Input: part model. Units: mm. Frame: model coordinates. Give positions to 0.01 mm unless a question says otherwise; leave off trailing zeros. Loops run counter-clockwise (first coordinate to the right, second up) from the corner with the lowest first, then second, coordinate; pieces in that order, holes last. Notation, with made-up numbers: (55, -5) - (77, -5) arc R31 cw to (77, 33) - close; hole circle Ø11 at (-38.5, 64). An arc over 180 degrees is marked (long way). One line per item, written item: value.
Autodesk Inventor part; units mm, degrees
ref_plane "YZ Plane" through (0, 0, 0) normal (1, 0, 0) x (0, 1, 0)
ref_plane "XZ Plane" through (0, 0, 0) normal (0, 1, 0) x (-1, 0, 0)
ref_plane "XY Plane" through (0, 0, 0) normal (0, 0, 1) x (1, 0, 0)
sketch "スケッチ2" plane through (0, 0, 0) normal (0, 0, 1) x (1, 0, 0)
  line L0 (-31.5, 10) -> (31.5, 10)
  line L1 (31.5, 10) -> (31.5, -10)
  line L2 (31.5, -10) -> (-31.5, -10)
  line L3 (-31.5, -10) -> (-31.5, 10)
  line L4 (0, 14) -> (0, -14) construction
  line L5 (-44.1, 0) -> (44.1, 0) construction
  point P0 (0, 0)
  dimension "d1" = 63
  dimension "d2" = 20
  dimension "d3" = 10
  dimension "d4" = 31.5
extrude "押し出し1" add sketch "スケッチ2" along normal blind 3
sketch "スケッチ3" plane through (0, 0, 3) normal (0, 0, 1) x (1, 0, 0)
  line L0 (-31.5, -10) -> (31.5, -10) construction
  line L1 (31.5, -10) -> (31.5, 10) construction
  line L2 (31.5, 10) -> (-31.5, 10) construction
  line L3 (-31.5, 10) -> (-31.5, -10) construction
  line L4 (-44.1, 0) -> (44.1, 0) construction
  point P0 (0, 0)
  point P1 (-21.5, 0)
  point P2 (1.5, 0)
  point P3 (21.5, 0)
  dimension "d7" = 10
  dimension "d8" = 10
  dimension "d9" = 20
hole "穴1" at (-21.5, 0, 3) at (1.5, 0, 3) at (21.5, 0, 3) direction (0, 0, -1) diameter 4.5 end through all
fillet "フィレット1" radius 2 4 edges at (-31.5, 10, 1.5) (31.5, 10, 1.5) (31.5, -10, 1.5) (-31.5, -10, 1.5)
equation "\"d3\" = 0.5 * d2"
equation "\"d4\" = 0.5 * d1"
properties part number "rocker_bogie_mount"
Item 1: Section B-B, the plane x = -21.5. Output: boundary loops of the cut face in (y, z), and give its area (3 significant figures).
Verdict:
outline: (-10, 0) - (-2.25, 0) - (-2.25, 3) - (-10, 3) - close; (2.25, 0) - (10, 0) - (10, 3) - (2.25, 3) - close
area: 46.5 mm^2
Item 2: Section A-A, the plane y = 0. Output: boundary loops of the cut face in (x, z), and give its area (4 significant figures).
Verdict:
outline: (-31.5, 0) - (-23.75, 0) - (-23.75, 3) - (-31.5, 3) - close; (-19.25, 0) - (-0.75, 0) - (-0.75, 3) - (-19.25, 3) - close; (3.75, 0) - (19.25, 0) - (19.25, 3) - (3.75, 3) - close; (23.75, 0) - (31.5, 0) - (31.5, 3) - (23.75, 3) - close
area: 148.5 mm^2
Item 3: Draft query along Y for faces 1 (the face through (-30.9, 9.43, 1.52)), 2 (the face through (3.696, 0.488, 1.479)), 3 (the face through (-31.5, 0, 1)). Return one class per face: pulls with the +Y half, pulls with the -Y half, needs draft (parallel to the pull), parting line crosses it, or undercut.
Verdict:
face 1: pulls with the +Y half
face 2: undercut
face 3: needs draft
Item 4: Section C-C, the plane z = 1.9. Output: boundary loops of the cut face in (x, y), and give its area (3 significant figures).
Verdict:
outline: (-31.5, -8) arc R2 ccw to (-29.5, -10) - (29.5, -10) arc R2 ccw to (31.5, -8) - (31.5, 8) arc R2 ccw to (29.5, 10) - (-29.5, 10) arc R2 ccw to (-31.5, 8) - close; hole circle Ø4.5 at (-21.5, 0); hole circle Ø4.5 at (1.5, 0); hole circle Ø4.5 at (21.5, 0)
area: 1,210 mm^2
Item 5: Material intervals for L1, parallel to X at y = 0, z = 0.7; L2, parallel to Y at x = 1.5, z = 0.9; L3, parallel to X at y = -1, z = 1.5, sorted ascending.
Verdict:
L1: x = -31.5 to -23.75, -19.25 to -0.75, 3.75 to 19.25, 23.75 to 31.5
L2: y = -10 to -2.25, 2.25 to 10
L3: x = -31.5 to -23.52, -19.48 to -0.52, 3.52 to 19.48, 23.52 to 31.5
